from build123d import *

# Parameters (mm, degrees)
SKETCH1_W            = 4
SKETCH1_H            = 80.5
BOSS_EXTRUDE1_DEPTH  = 71
BOSS_EXTRUDE2_START  = -4
BOSS_EXTRUDE2_DEPTH  = 4
BOSS_EXTRUDE3_DEPTH  = 34.2
CUT_EXTRUDE1_DEPTH   = 13
CUT_EXTRUDE2_DEPTH   = 13
SKETCH6_R            = 1.7
CUT_EXTRUDE3_DEPTH   = 13
SKETCH7_R            = 3.25
CUT_EXTRUDE4_DEPTH   = 2.5
BOSS_EXTRUDE4_DEPTH  = 44.5
SKETCH10_W           = 46.002383675
SKETCH10_H           = 61.711229379
CUT_EXTRUDE5_DEPTH   = 42
FILLET1_R            = 18
BOSS_EXTRUDE5_DEPTH  = 4
FILLET3_R            = 16.2
FILLET4_R            = 14
CUT_EXTRUDE6_DEPTH   = 10.6
BOSS_EXTRUDE6_START  = 4
BOSS_EXTRUDE6_DEPTH  = 4
CUT_EXTRUDE7_DEPTH   = 148
BOSS_EXTRUDE7_DEPTH  = 3
CUT_EXTRUDE8_DEPTH   = 14
SKETCH17_R           = 2.25
CUT_EXTRUDE9_DEPTH   = 14
SKETCH18_W           = 25
SKETCH18_H           = 92.2
BOSS_EXTRUDE8_DEPTH  = 4
SKETCH19_W           = 4
SKETCH19_H           = 92.2
BOSS_EXTRUDE9_DEPTH  = 4
SKETCH20_R           = 5.25
CUT_EXTRUDE10_DEPTH  = 4
SKETCH21_W           = 33
SKETCH21_H           = 92.2
CUT_EXTRUDE11_DEPTH  = 0.6
SKETCH22_R           = 5.25
CUT_EXTRUDE12_DEPTH  = 3.4
BOSS_EXTRUDE10_DEPTH = 40
SKETCH24_R           = 6.4
CUT_EXTRUDE13_DEPTH  = 3.4
BOSS_EXTRUDE11_DEPTH = 15
SKETCH26_W           = 10
SKETCH26_H           = 1.5
BOSS_EXTRUDE12_DEPTH = 15
CUT_EXTRUDE14_DEPTH  = 15
SKETCH28_W           = 33
SKETCH28_H           = 3.4
CUT_EXTRUDE15_DEPTH  = 1


with BuildPart() as part:
    # Sketch1 → Boss-Extrude1 (new body)
    with BuildSketch(Plane.XY):
        with Locations((2, 40.25)):
            Rectangle(SKETCH1_W, SKETCH1_H)
        with BuildLine():
            Line((0, 80.5), (4, 80.5))
            ThreePointArc((4, 80.5), (16.5, 93), (29, 80.5))
            Line((29, 80.5), (33, 80.5))
            ThreePointArc((33, 80.5), (16.5, 97), (0, 80.5))
        make_face()
        with Locations((31, 40.25)):
            Rectangle(SKETCH1_W, SKETCH1_H)
    extrude(amount=BOSS_EXTRUDE1_DEPTH)

    # Sketch2 → Boss-Extrude2 (add)
    with BuildSketch(Plane.XY.offset(71).offset(BOSS_EXTRUDE2_START)):
        with BuildLine():
            Line((33, 48.5), (0, 48.5))
            Line((0, 48.5), (0, 80.5))
            ThreePointArc((0, 80.5), (16.5, 97), (33, 80.5))
            Line((33, 80.5), (33, 48.5))
        make_face()
    extrude(amount=BOSS_EXTRUDE2_DEPTH)

    # Sketch3 → Boss-Extrude3 (add)
    with BuildSketch(Plane(origin=(0, 0, 67), x_dir=(-1, 0, 0), z_dir=(0, 0, -1))):
        Polygon((-33, 0), (-33, 48.5), (-29, 48.5), (-4, 48.5), (0, 48.5), (0, 0), (-3.837905566, 0), (-4, 44.5), (-29, 44.5), (-29.162094434, 0), align=None)
    extrude(amount=-BOSS_EXTRUDE3_DEPTH)

    # Sketch4 → Cut-Extrude1 (cut)
    with BuildSketch(Plane(origin=(0, 0, 0), x_dir=(-1, 0, 0), z_dir=(0, 0, -1))):
        with BuildLine():
            Line((-4, 80.5), (-4, 0))
            Line((-4, 0), (0, 0))
            Line((0, 0), (0, 80.5))
            ThreePointArc((0, 80.5), (-16.5, 97), (-33, 80.5))
            Line((-33, 80.5), (-33, 0))
            Line((-33, 0), (-29, 0))
            Line((-29, 0), (-29, 80.5))
            ThreePointArc((-29, 80.5), (-16.5, 93), (-4, 80.5))
        make_face()
    extrude(amount=-CUT_EXTRUDE1_DEPTH, mode=Mode.SUBTRACT)

    # Sketch5 → Cut-Extrude2 (cut)
    with BuildSketch(Plane.XY.offset(71)):
        with BuildLine():
            ThreePointArc((26.5, 80.5), (16.5, 90.5), (6.5, 80.5))
            Line((6.5, 80.5), (26.5, 80.5))
        make_face()
        with BuildLine():
            Line((26.5, 80.5), (6.5, 80.5))
            ThreePointArc((6.5, 80.5), (16.5, 70.5), (26.5, 80.5))
        make_face()
    extrude(amount=-CUT_EXTRUDE2_DEPTH, mode=Mode.SUBTRACT)

    # Sketch6 → Cut-Extrude3 (cut)
    with BuildSketch(Plane.XY.offset(71)):
        with Locations((6.5, 70.5)):
            Circle(SKETCH6_R)
        with BuildLine():
            ThreePointArc((28.2, 70.5), (26.5, 72.2), (24.8, 70.5))
            Line((24.8, 70.5), (28.2, 70.5))
        make_face()
        with BuildLine():
            Line((28.2, 70.5), (24.8, 70.5))
            ThreePointArc((24.8, 70.5), (26.5, 68.8), (28.2, 70.5))
        make_face()
    extrude(amount=-CUT_EXTRUDE3_DEPTH, mode=Mode.SUBTRACT)

    # Sketch7 → Cut-Extrude4 (cut)
    with BuildSketch(Plane.XY.offset(71)):
        with Locations((6.5, 70.5)):
            Circle(SKETCH7_R)
        with Locations((26.5, 70.5)):
            Circle(SKETCH7_R)
    extrude(amount=-CUT_EXTRUDE4_DEPTH, mode=Mode.SUBTRACT)

    # Sketch9 → Boss-Extrude4 (add)
    with BuildSketch(Plane.XZ):
        Polygon((29.162094434, 101.2), (29.162094434, 71), (29, 71), (29, 120), align=None)
        Polygon((4, 120), (3.837905566, 101.2), (3.837905566, 71), (4, 71), align=None)
    extrude(amount=-BOSS_EXTRUDE4_DEPTH)

    # Sketch10 → Cut-Extrude5 (cut)
    with BuildSketch(Plane.XY.offset(101.2)):
        with Locations((17.24268837, 24.291112106)):
            Rectangle(SKETCH10_W, SKETCH10_H)
    extrude(amount=CUT_EXTRUDE5_DEPTH, mode=Mode.SUBTRACT)

    # Fillet1
    fillet1_edges = [part.edges().sort_by_distance(p)[0] for p in [
        (16.5, 48.5, 71),
        (16.5, 44.5, 67),
    ]]
    fillet(fillet1_edges, radius=FILLET1_R)

    # Sketch11 → Boss-Extrude5 (add)
    with BuildSketch(Plane.XY.offset(101.2)):
        Polygon((29, 0), (4, 0), (0, 0), (0, 48.5), (33, 48.5), (33, 0), align=None)
    extrude(amount=BOSS_EXTRUDE5_DEPTH)

    # Fillet3
    fillet3_edges = [part.edges().sort_by_distance(p)[0] for p in [
        (16.5, 48.5, 105.2),
    ]]
    fillet(fillet3_edges, radius=FILLET3_R - 0.0001)  # a hair under: the kernel refuses the full size

    # Fillet4
    fillet4_edges = [part.edges().sort_by_distance(p)[0] for p in [
        (16.5, 44.5, 101.2),
    ]]
    fillet(fillet4_edges, radius=FILLET4_R)

    # Sketch12 → Cut-Extrude6 (cut)
    with BuildSketch(Plane.XZ):
        Polygon((4, 13), (4, 101.2), (29, 101.2), (29, 13), (33, 13), (33, 105.2), (0, 105.2), (0, 13), align=None)
    extrude(amount=-CUT_EXTRUDE6_DEPTH, mode=Mode.SUBTRACT)

    # Sketch13 → Boss-Extrude6 (add)
    with BuildSketch(Plane(origin=(0, 0, 13), x_dir=(-1, 0, 0), z_dir=(0, 0, -1)).offset(BOSS_EXTRUDE6_START)):
        with BuildLine():
            Line((-33, 80.5), (-33, 10.6))
            Line((-33, 10.6), (-29, 10.6))
            Line((-29, 10.6), (-29, 80.5))
            ThreePointArc((-29, 80.5), (-16.5, 93), (-4, 80.5))
            Line((-4, 80.5), (-4, 10.6))
            Line((-4, 10.6), (0, 10.6))
            Line((0, 10.6), (0, 80.5))
            ThreePointArc((0, 80.5), (-16.5, 97), (-33, 80.5))
        make_face()
    extrude(amount=-BOSS_EXTRUDE6_DEPTH)

    # Sketch14 → Cut-Extrude7 (cut)
    with BuildSketch(Plane(origin=(0, 0, 13), x_dir=(-1, 0, 0), z_dir=(0, 0, -1))):
        with BuildLine():
            Line((-29, 10.6), (-4, 10.6))
            Line((-4, 10.6), (0, 10.6))
            Line((0, 10.6), (0, 80.5))
            ThreePointArc((0, 80.5), (-16.5, 97), (-33, 80.5))
            Line((-33, 80.5), (-33, 10.6))
            Line((-33, 10.6), (-29, 10.6))
        make_face()
    extrude(amount=-CUT_EXTRUDE7_DEPTH, mode=Mode.SUBTRACT)

    # Sketch16 → Cut-Extrude8 (cut)
    with BuildSketch(Plane(origin=(0, 0, 9), x_dir=(-1, 0, 0), z_dir=(0, 0, -1))):
        with BuildLine():
            Line((-33, 80.5), (-33, 10.6))
            Line((-33, 10.6), (-29, 10.6))
            Line((-29, 10.6), (-29, 80.5))
            ThreePointArc((-29, 80.5), (-16.5, 93), (-4, 80.5))
            Line((-4, 80.5), (-4, 10.6))
            Line((-4, 10.6), (0, 10.6))
            Line((0, 10.6), (0, 80.5))
            ThreePointArc((0, 80.5), (-16.5, 97), (-33, 80.5))
        make_face()
    extrude(amount=-CUT_EXTRUDE8_DEPTH, mode=Mode.SUBTRACT)


with BuildPart() as body_2:
    # Sketch15 → Boss-Extrude7 (new body)
    with BuildSketch(Plane.XY.offset(13)):
        with BuildLine():
            Line((4, 10.6), (29, 10.6))
            Line((29, 10.6), (29, 80.5))
            ThreePointArc((29, 80.5), (16.5, 93), (4, 80.5))
            Line((4, 80.5), (4, 10.6))
        make_face()
    extrude(amount=BOSS_EXTRUDE7_DEPTH)

    # Sketch17 → Cut-Extrude9 (cut)
    with BuildSketch(Plane(origin=(0, 0, 13), x_dir=(-1, 0, 0), z_dir=(0, 0, -1))):
        with Locations((-24, 72)):
            Circle(SKETCH17_R)
        with Locations((-9, 72)):
            Circle(SKETCH17_R)
    extrude(amount=-CUT_EXTRUDE9_DEPTH, mode=Mode.SUBTRACT)

    # Sketch18 → Boss-Extrude8 (add)
    with BuildSketch(Plane.XZ.offset(-10.6)):
        with Locations((16.5, -30.1)):
            Rectangle(SKETCH18_W, SKETCH18_H)
    extrude(amount=BOSS_EXTRUDE8_DEPTH)

    # Sketch19 → Boss-Extrude9 (add)
    with BuildSketch(Plane.XZ.offset(-6.6)):
        with Locations((2, -30.1)):
            Rectangle(SKETCH19_W, SKETCH19_H)
        with Locations((31, -30.1)):
            Rectangle(SKETCH19_W, SKETCH19_H)
    extrude(amount=-BOSS_EXTRUDE9_DEPTH)

    # Sketch20 → Cut-Extrude10 (cut)
    with BuildSketch(Plane.XZ.offset(-6.6)):
        with Locations(Location((16.5, -10.7, 0), (0, 0, 270))):
            Circle(SKETCH20_R)
    extrude(amount=-CUT_EXTRUDE10_DEPTH, mode=Mode.SUBTRACT)

    # Sketch21 → Cut-Extrude11 (cut)
    with BuildSketch(Plane.XZ.offset(-6.6)):
        with Locations((16.5, -30.1)):
            Rectangle(SKETCH21_W, SKETCH21_H)
    extrude(amount=-CUT_EXTRUDE11_DEPTH, mode=Mode.SUBTRACT)

    # Sketch22 → Cut-Extrude12 (cut)
    with BuildSketch(Plane.XZ.offset(-7.2)):
        with Locations(Location((16.5, 1.3, 0), (0, 0, 270))):
            Circle(SKETCH22_R)
    extrude(amount=-CUT_EXTRUDE12_DEPTH, mode=Mode.SUBTRACT)

    # Sketch23 → Boss-Extrude10 (add)
    with BuildSketch(Plane.XZ.offset(-7.2)):
        with BuildLine():
            ThreePointArc((16.5, 10.35), (8.6, 2.45), (16.5, -5.45))
            Line((16.5, -5.45), (16.5, -3.95))
            ThreePointArc((16.5, -3.95), (10.1, 2.45), (16.5, 8.85))
            Line((16.5, 8.85), (16.5, 10.35))
        make_face()
        with BuildLine():
            Line((16.5, -3.95), (16.5, -5.45))
            ThreePointArc((16.5, -5.45), (22.086143571, -3.136143571), (24.4, 2.45))
            ThreePointArc((24.4, 2.45), (22.086143571, 8.036143571), (16.5, 10.35))
            Line((16.5, 10.35), (16.5, 8.85))
            ThreePointArc((16.5, 8.85), (21.0254834, 6.9754834), (22.9, 2.45))
            ThreePointArc((22.9, 2.45), (21.0254834, -2.0754834), (16.5, -3.95))
        make_face()
    extrude(amount=BOSS_EXTRUDE10_DEPTH)

    # Sketch24 → Cut-Extrude13 (cut)
    with BuildSketch(Plane.XZ.offset(-7.2)):
        with Locations(Location((16.5, 2.45, 0), (0, 0, 270))):
            Circle(SKETCH24_R)
    extrude(amount=-CUT_EXTRUDE13_DEPTH, mode=Mode.SUBTRACT)

    # Sketch25 → Boss-Extrude11 (add)
    with BuildSketch(Plane(origin=(0, 10.6, 0), x_dir=(1, 0, 0), z_dir=(0, 1, 0))):
        Polygon((26.5, 72.7), (6.5, 72.7), (6.5, 74.7), (16.5, 74.7), (26.5, 74.7), align=None)
    extrude(amount=BOSS_EXTRUDE11_DEPTH)

    # Sketch26 → Boss-Extrude12 (add)
    with BuildSketch(Plane(origin=(0, 10.6, 0), x_dir=(1, 0, 0), z_dir=(0, 1, 0))):
        with Locations((16.5, 75.45)):
            Rectangle(SKETCH26_W, SKETCH26_H)
    extrude(amount=BOSS_EXTRUDE12_DEPTH)

    # Sketch27 → Cut-Extrude14 (cut)
    with BuildSketch(Plane(origin=(0, 10.6, 0), x_dir=(1, 0, 0), z_dir=(0, 1, 0))):
        Polygon((6.5, 72.7), (26.5, 72.7), (26.5, 74.7), (21.5, 74.7), (21.5, 76.2), (11.5, 76.2), (11.5, 74.7), (6.5, 74.7), align=None)
    extrude(amount=CUT_EXTRUDE14_DEPTH, mode=Mode.SUBTRACT)

    # Sketch28 → Cut-Extrude15 (cut)
    with BuildSketch(Plane(origin=(0, 0, -76.2), x_dir=(-1, 0, 0), z_dir=(0, 0, -1))):
        with Locations((-16.5, 8.9)):
            Rectangle(SKETCH28_W, SKETCH28_H)
    extrude(amount=-CUT_EXTRUDE15_DEPTH, mode=Mode.SUBTRACT)


solid = body_2.part
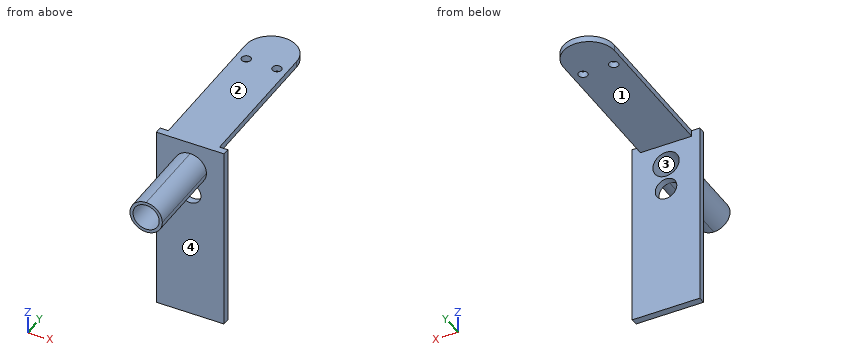
Check sheet for the modelled part. Datum: model origin and axes. Units: mm. Face numbers are marked on the shaded views. A direction names the side the tool comes from. Give positions to 0.01 mm unless a question says otherwise; leave off trailing zeros. Loops run counter-clockwise (first coordinate to the right, second up) from the corner with the lowest first, then second, coordinate; pieces in that order, holes last. Notation, with made-up numbers: M 30,65.25 L 58,65.25 A16 cw 58,95.25 Z; hole C 29,-30 d1. An arc over 180 degrees is marked long. Return JSON: item names as keys, results as strings. Group by question number.
1. Cross-section at A-A on z = -10.7. Record the boundary of the cut face in (x, y).
2. Go/stop test with flat-tipped pins: pin 1 (1.5 mm diameter, centred on y = 46, z = 15, fed in from +X); pin 2 (4 mm diameter, centred on x = 29.5, z = -43.5, fed in from +Y); pin 3 (7 mm diameter, centred on x = 24, y = 72, fed in from -Z); pin 4 (4 mm diameter, centred on x = 9, y = 72, fed in from +Z). Record where each tip stops, or that it passes through.
3. Cross-section at C-C on y = 5. Record the boundary of the cut face in (x, z), plus the area to 3 significant figures.
4. Tool access check on the marked faces 1 and 2. Record the directions out of +Z, -Z, +X, -X, +Y, -Y that give a thin tool (end or side, any length) a straight path to the whole face; none if there is none.
5. Mould release check, pull along X, two halves, no side actions. Record for the marked faces 3 and 4: released by +X, released by -X, zero draft, split by the parting line, or undercut.
6. Cross-section at D-D on z = 6.5. Record the boundary of the cut face in (x, y).
7. Thickness scan on L1, parallel to Z at x = 16.5, y = 8.5; L2, parallel to Z at x = 16, y = -22; L3, parallel to X at y = -10, z = 2.45. Record the ranges inside material, lowest first.
8. Cross-section at B-B on y = 72. Record the boundary of the cut face in (x, z), plus the area to 3 significant figures.
Return value:
{
 "1": {"outline": "M 0,7.2 L 11.25,7.2 L 11.25,10.6 L 0,10.6 Z; M 21.75,7.2 L 33,7.2 L 33,10.6 L 21.75,10.6 Z"},
 "2": {"pin 1": "x = 29", "pin 2": "y = 10.6", "pin 3": "z = 13", "pin 4": "through"},
 "3": {"outline": "C 16.5,2.45 d15.8; hole C 16.5,2.45 d12.8", "area": "67.4 mm^2"},
 "4": {"face 1": "-Z, +X, -X, +Y", "face 2": "+Z, +X, -X, +Y, -Y"},
 "5": {"face 3": "undercut", "face 4": "zero draft"},
 "6": {"outline": "M 0,7.2 L 9.72,7.2 L 9.72,-32.8 L 11.54,-32.8 L 11.54,10.6 L 0,10.6 Z; M 21.46,-32.8 L 23.28,-32.8 L 23.28,7.2 L 33,7.2 L 33,10.6 L 21.46,10.6 Z"},
 "7": {"L1": "-75.2 to -15.95, -5.45 to -3.95, 8.85 to 16", "L2": "-5.43 to -3.93, 8.83 to 10.33", "L3": "8.6 to 10.1, 22.9 to 24.4"},
 "8": {"outline": "M 4,13 L 6.75,13 L 6.75,16 L 4,16 Z; M 11.25,13 L 21.75,13 L 21.75,16 L 11.25,16 Z; M 26.25,13 L 29,13 L 29,16 L 26.25,16 Z", "area": "48.0 mm^2"}
}
